For this review, take the finished solid that the model builds, in its own axes (mm). A direction names the side the tool comes from. Coordinates: 2 decimals unless noted, no trailing zeros. Loops run counter-clockwise (first coordinate to the right, second up) from the corner with the lowest first, then second, coordinate; pieces in that order, holes last. Notation, with made-up numbers: (-36, -17.75) -> (-7, -17.75) arc R13 ccw to (-7, -11.75) -> close; hole circle Ø10 at (69, 35.5). An arc over 180 degrees is marked (long way). Use a Markdown table: item, result.
from build123d import *

# Parameters (mm, degrees)
SKETCH1_W           = 381
SKETCH1_H           = 50.8
BOSS_EXTRUDE1_DEPTH = 2.794
SKETCH2_W           = 381
SKETCH2_H           = 2.794
BOSS_EXTRUDE2_DEPTH = 48.006
SKETCH3_R           = 8
CUT_EXTRUDE1_DEPTH  = 2.794
SKETCH4_W           = 139.7
SKETCH4_H           = 48.006
CUT_EXTRUDE2_DEPTH  = 2.794


with BuildPart() as part:
    # Sketch1 → Boss-Extrude1 (new body)
    with BuildSketch(Plane(origin=(0, 0, 0), x_dir=(1, 0, 0), z_dir=(0, 1, 0))):
        Rectangle(SKETCH1_W, SKETCH1_H)
    extrude(amount=BOSS_EXTRUDE1_DEPTH)

    # Sketch2 → Boss-Extrude2 (add)
    with BuildSketch(Plane(origin=(0, 2.794, 0), x_dir=(1, 0, 0), z_dir=(0, 1, 0))):
        with Locations((0, -24.003)):
            Rectangle(SKETCH2_W, SKETCH2_H)
    extrude(amount=BOSS_EXTRUDE2_DEPTH)

    # Sketch3 → Cut-Extrude1 (cut)
    with BuildSketch(Plane.XY.offset(25.4)):
        with Locations((0, 25.4)):
            Circle(SKETCH3_R)
    extrude(amount=-CUT_EXTRUDE1_DEPTH, mode=Mode.SUBTRACT)

    # Sketch4 → Cut-Extrude2 (cut)
    with BuildSketch(Plane.XY.offset(25.4)):
        with Locations((-120.65, 26.797)):
            Rectangle(SKETCH4_W, SKETCH4_H)
        with Locations((120.65, 26.797)):
            Rectangle(SKETCH4_W, SKETCH4_H)
    extrude(amount=-CUT_EXTRUDE2_DEPTH, mode=Mode.SUBTRACT)


solid = part.part
(1) Take a section at D-D on x = 151. Write out the cut boundary in (y, z).
Found:
| item | result |
|---|---|
| outline | (0, -25.4) -> (2.79, -25.4) -> (2.79, 25.4) -> (0, 25.4) -> close |
(2) Take a section at C-C on z = -18.5. Write out the cut boundary in (x, y), plus the area to 3 significant figures.
Found:
| item | result |
|---|---|
| outline | (-190.5, 0) -> (190.5, 0) -> (190.5, 2.79) -> (-190.5, 2.79) -> close |
| area | 1,060 mm^2 |
(3) For line 1 along Y through (x, z) = (0, 24.4); line 2 along Y through (x, z) = (-62.5, -0.5); line 3 along Z through (x, y) = (-10.5, 30.5), list the stretches that pass through material, from the lowest coordinate up.
Found:
| item | result |
|---|---|
| line 1 | y = 0 to 17.4, 33.4 to 50.8 |
| line 2 | y = 0 to 2.79 |
| line 3 | z = 22.61 to 25.4 |
(4) Take a section at A-A on x = 0. Write out the cut boundary in (y, z), plus the area to 3 significant figures.
Found:
| item | result |
|---|---|
| outline | (0, -25.4) -> (2.79, -25.4) -> (2.79, 22.61) -> (17.4, 22.61) -> (17.4, 25.4) -> (0, 25.4) -> close; (33.4, 22.61) -> (50.8, 22.61) -> (50.8, 25.4) -> (33.4, 25.4) -> close |
| area | 231 mm^2 |
(5) For faces 1 (the face through (-1, 16, 22.606)), 2 (the face through (-3, 14, 25.4)), list the 3-axis set-ups (+Z, -Z, +X, -X, +Y, -Y) from which the entire face can be reached by the end or side of a thin tool; tool diameter is ignored.
Found:
| item | result |
|---|---|
| face 1 | -Z, +X, -X, +Y |
| face 2 | +Z, +X, -X, +Y, -Y |
(6) For pin 1 Ø10 at (x, y) = (-19, 42) entering from -Z; pin 2 Ø13 at (x, y) = (0, 25.4) entering from +Z; pin 3 Ø2 at (y, z) = (30, 23.5) entering from +X; pin 4 Ø2 at (y, z) = (38.5, 24) entering from -X, all flat-tipped, find the tip position at first contact; note any pin that passes through.
Found:
| item | result |
|---|---|
| pin 1 | stops at z = 22.61 |
| pin 2 | passes through |
| pin 3 | stops at x = 50.8 |
| pin 4 | stops at x = -50.8 |
(7) Mouldability with a two-part tool opening along X and no side actions: class faces 3 (the face through (-1.73, 17.59, 24.02)), 4 (the face through (-3, 0, 0)) as pulls with the +X half, pulls with the -X half, needs draft (parallel to the pull), parting line crosses it, or undercut.
Found:
| item | result |
|---|---|
| face 3 | undercut |
| face 4 | needs draft |
(8) Take a section at B-B on y = 25.4. Write out the cut boundary in (x, z).
Found:
| item | result |
|---|---|
| outline | (-50.8, 22.61) -> (-8, 22.61) -> (-8, 25.4) -> (-50.8, 25.4) -> close; (8, 22.61) -> (50.8, 22.61) -> (50.8, 25.4) -> (8, 25.4) -> close |
